from build123d import *

# Parameters (mm, degrees)
BOSS_EXTRUDE1_DEPTH = 10
CUT_EXTRUDE1_DEPTH  = 11
SKETCH3_R           = 1.75
CUT_EXTRUDE2_DEPTH  = 119.9


with BuildPart() as part:
    # Sketch1 → Boss-Extrude1 (new body)
    with BuildSketch(Plane.XY):
        Polygon((0, 0), (0, 5), (-10, 5), (-10, 10), (0, 10), (0, 119), (-10, 119), (-10, 124), (10, 124), (10, 0), align=None)
    extrude(amount=-BOSS_EXTRUDE1_DEPTH)

    # Sketch2 → Cut-Extrude1 (cut, through all)
    with BuildSketch(Plane.XY):
        Polygon((-10, 10), (-10, 5), (0, 5), (0, 0), (0.1, 0), (0.1, 5.1), (-9.9, 5.1), (-9.9, 10), align=None)
        Polygon((-10, 124), (-10, 119), (0, 119), (0, 113.9), (0.1, 113.9), (0.1, 119.1), (-9.9, 119.1), (-9.9, 124), align=None)
    extrude(amount=-CUT_EXTRUDE1_DEPTH, mode=Mode.SUBTRACT)

    # Sketch3 → Cut-Extrude2 (cut, through all)
    with BuildSketch(Plane.XZ.offset(-5.1)):
        with Locations((-5, -5)):
            Circle(SKETCH3_R)
    extrude(amount=-CUT_EXTRUDE2_DEPTH, mode=Mode.SUBTRACT)


solid = part.part
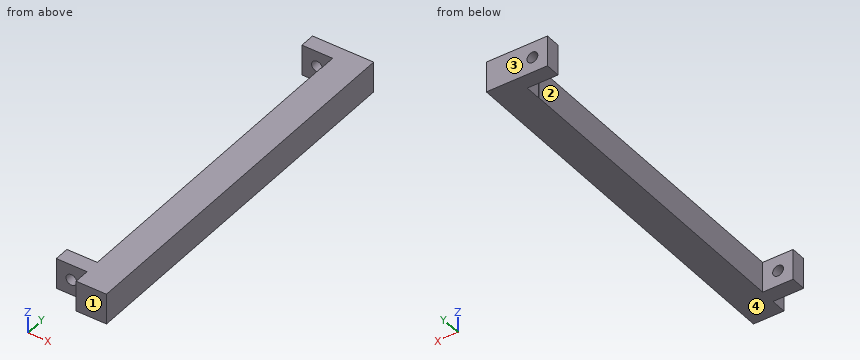
Work out the finished part from the listing and answer in its coordinate system (mm). Face numbers are marked on the shaded views. Round coordinates to 2 decimals unless told otherwise and drop trailing zeros. Write each loop counter-clockwise with the first axis right and the second up, starting at its lowest first coordinate (ties: lowest second). Pieces come first, ordered by that corner, then holes. Notation, with made-up numbers: (16, 14.5) - (32, 14.5) arc R12 ccw to (32, 24.5) - close; hole circle Ø11 at (59.5, 16). An arc over 180 degrees is marked (long way). Answer in a Markdown table with one row per item. Add a question column.
1. A cutting plane is placed at B-B, the plane x = -2. Determine the outline of the cut face in (y, z), and give its area (3 significant figures).
2. Find the intervals of material crossed by line 1 along Z through (x, y) = (-5, 7.55); line 2 along X through (y, z) = (82.5, -4.25); line 3 along Y through (x, z) = (-1.25, -9), in increasing order. Write a range as from..to.
3. A cutting plane is placed at C-C, the plane y = 49.5. Determine the outline of the cut face in (x, z), and give its area (3 significant figures).
4. Given pin 1 (4 mm diameter, centred on x = -6.5, z = -5, fed in from -Y); pin 2 (2 mm diameter, centred on y = 40, z = -9, fed in from -X); pin 3 (1.5 mm diameter, centred on y = 4, z = -3, fed in from -X), each flat-ended and moving along its own axis, determine where each tip first touches the part or whether it passes through.
5. A cutting plane is placed at A-A, the plane z = -5. Determine the outline of the cut face in (x, y), and give its area (3 significant figures).
6. The mould has two halves that part along Y. Classify the marked faces 1, 2, 3 and 4: +Y half, -Y half, draft (parallel to the pull), parting line (faces both ways), or undercut.
Worked out:
| question | item | result |
|---|---|---|
| 1 | outline | (5.1, -10) - (10, -10) - (10, 0) - (5.1, 0) - close; (119.1, -10) - (124, -10) - (124, 0) - (119.1, 0) - close |
| 1 | area | 98.0 mm^2 |
| 2 | line 1 | -10..-6.75, -3.25..0 |
| 2 | line 2 | 0..10 |
| 2 | line 3 | 5.1..10, 119.1..124 |
| 3 | outline | (0, -10) - (10, -10) - (10, 0) - (0, 0) - close |
| 3 | area | 100 mm^2 |
| 4 | pin 1 | y = 5.1 |
| 4 | pin 2 | x = 0 |
| 4 | pin 3 | x = 0.1 |
| 5 | outline | (-9.9, 5.1) - (-6.75, 5.1) - (-6.75, 10) - (-9.9, 10) - close; (-9.9, 119.1) - (-6.75, 119.1) - (-6.75, 124) - (-9.9, 124) - close; (-3.25, 5.1) - (0.1, 5.1) - (0.1, 0) - (10, 0) - (10, 124) - (-3.25, 124) - (-3.25, 119.1) - (0.1, 119.1) - (0.1, 113.9) - (0, 113.9) - (0, 10) - (-3.25, 10) - close |
| 5 | area | 1,300 mm^2 |
| 6 | face 1 | -Y half |
| 6 | face 2 | undercut |
| 6 | face 3 | +Y half |
| 6 | face 4 | draft |
